The model under review builds one solid part; all positions refer to its coordinate system, in mm. A direction names the side the tool comes from. Give positions to 0.01 mm unless a question says otherwise; leave off trailing zeros. Loops run counter-clockwise (first coordinate to the right, second up) from the corner with the lowest first, then second, coordinate; pieces in that order, holes last. Notation, with made-up numbers: M -15.5,-21.5 L 37.5,-21.5 A12 cw 37.5,-0.5 Z; hole C -31,77 d4. An arc over 180 degrees is marked long. Return JSON: item names as keys, results as strings.
```python
from build123d import *

# Parameters (mm, degrees)
F0_R     = 11
F2_DEPTH = 2.5
F1_R     = 3.1
F1_R_2   = 1.25
F1_R_3   = 1
F3_DEPTH = 2.501
F4_R     = 2.2
F5_DEPTH = 1.8
F6_R     = 6.3
F7_DEPTH = 0.8
F8_DEPTH = 0.8
F9_DEPTH = 3.301


with BuildPart() as f2:
    # F0 (on Front) → F2 (new body)
    with BuildSketch(Plane.XZ):
        Circle(F0_R)
    extrude(amount=F2_DEPTH)

    # F1 (on Front) → F3 (cut, through all)
    with BuildSketch(Plane.XZ):
        Circle(F1_R)
        with Locations((-6.5, 0)):
            Circle(F1_R_2)
        with Locations((-6.363961, 6.363961)):
            Circle(F1_R_3)
        with Locations((-6.363961, -6.363961)):
            Circle(F1_R_3)
        with Locations((6.363961, -6.363961)):
            Circle(F1_R_3)
        with Locations((6.363961, 6.363961)):
            Circle(F1_R_3)
        with Locations((6.5, 0)):
            Circle(F1_R_2)
        with BuildLine():
            ThreePointArc((1.1, -5), (0, -3.9), (-1.1, -5))
            Line((-1.1, -5), (-1.1, -6.133975))
            ThreePointArc((-1.1, -6.133975), (-1.4, -7), (-1.1, -7.866025))
            Line((-1.1, -7.866025), (-1.1, -8.5))
            ThreePointArc((-1.1, -8.5), (0, -9.6), (1.1, -8.5))
            Line((1.1, -8.5), (1.1, -7.866025))
            ThreePointArc((1.1, -7.866025), (1.4, -7), (1.1, -6.133975))
            Line((1.1, -6.133975), (1.1, -5))
        make_face()
        with BuildLine():
            Line((-1.1, 8.5), (-1.1, 7.866025))
            ThreePointArc((-1.1, 7.866025), (-1.4, 7), (-1.1, 6.133975))
            Line((-1.1, 6.133975), (-1.1, 5))
            ThreePointArc((-1.1, 5), (0, 3.9), (1.1, 5))
            Line((1.1, 5), (1.1, 6.133975))
            ThreePointArc((1.1, 6.133975), (1.4, 7), (1.1, 7.866025))
            Line((1.1, 7.866025), (1.1, 8.5))
            ThreePointArc((1.1, 8.5), (0, 9.6), (-1.1, 8.5))
        make_face()
    extrude(amount=F3_DEPTH, mode=Mode.SUBTRACT)

    # F4 (on face) → F5 (cut)
    with BuildSketch(Plane.XZ.offset(2.5)):
        with Locations((-6.5, 0)):
            Circle(F4_R)
        with Locations((6.5, 0)):
            Circle(F4_R)
        with BuildLine():
            Line((1.8, 4.4), (1.8, 5.265065))
            ThreePointArc((1.8, 5.265065), (2.499967, 7.01284), (1.782084, 8.753333))
            ThreePointArc((1.782084, 8.753333), (0, 10.3), (-1.782084, 8.753333))
            ThreePointArc((-1.782084, 8.753333), (-2.499967, 7.01284), (-1.8, 5.265065))
            Line((-1.8, 5.265065), (-1.8, 4.4))
            ThreePointArc((-1.8, 4.4), (-1.634926, 3.646995), (-1.169981, 3.032102))
            ThreePointArc((-1.169981, 3.032102), (0, 3.25), (1.169981, 3.032102))
            ThreePointArc((1.169981, 3.032102), (1.634926, 3.646995), (1.8, 4.4))
        make_face()
        with BuildLine():
            Line((-1.8, -4.4), (-1.8, -5.265065))
            ThreePointArc((-1.8, -5.265065), (-2.499967, -7.01284), (-1.782084, -8.753333))
            ThreePointArc((-1.782084, -8.753333), (0, -10.3), (1.782084, -8.753333))
            ThreePointArc((1.782084, -8.753333), (2.499967, -7.01284), (1.8, -5.265065))
            Line((1.8, -5.265065), (1.8, -4.4))
            ThreePointArc((1.8, -4.4), (1.634926, -3.646995), (1.169981, -3.032102))
            ThreePointArc((1.169981, -3.032102), (0, -3.25), (-1.169981, -3.032102))
            ThreePointArc((-1.169981, -3.032102), (-1.634926, -3.646995), (-1.8, -4.4))
        make_face()
    extrude(amount=-F5_DEPTH, mode=Mode.SUBTRACT)

    # F6 (on face) → F7 (join)
    with BuildSketch(Plane.XZ.offset(2.5)):
        Circle(F6_R)
    extrude(amount=F7_DEPTH)

    # F4 (on face) → F8 (cut)
    with BuildSketch(Plane.XZ.offset(2.5)):
        with Locations((-6.5, 0)):
            Circle(F4_R)
        with Locations((6.5, 0)):
            Circle(F4_R)
        with BuildLine():
            Line((1.8, 4.4), (1.8, 5.265065))
            ThreePointArc((1.8, 5.265065), (2.499967, 7.01284), (1.782084, 8.753333))
            ThreePointArc((1.782084, 8.753333), (0, 10.3), (-1.782084, 8.753333))
            ThreePointArc((-1.782084, 8.753333), (-2.499967, 7.01284), (-1.8, 5.265065))
            Line((-1.8, 5.265065), (-1.8, 4.4))
            ThreePointArc((-1.8, 4.4), (-1.634926, 3.646995), (-1.169981, 3.032102))
            ThreePointArc((-1.169981, 3.032102), (0, 3.25), (1.169981, 3.032102))
            ThreePointArc((1.169981, 3.032102), (1.634926, 3.646995), (1.8, 4.4))
        make_face()
        with BuildLine():
            Line((-1.8, -4.4), (-1.8, -5.265065))
            ThreePointArc((-1.8, -5.265065), (-2.499967, -7.01284), (-1.782084, -8.753333))
            ThreePointArc((-1.782084, -8.753333), (0, -10.3), (1.782084, -8.753333))
            ThreePointArc((1.782084, -8.753333), (2.499967, -7.01284), (1.8, -5.265065))
            Line((1.8, -5.265065), (1.8, -4.4))
            ThreePointArc((1.8, -4.4), (1.634926, -3.646995), (1.169981, -3.032102))
            ThreePointArc((1.169981, -3.032102), (0, -3.25), (-1.169981, -3.032102))
            ThreePointArc((-1.169981, -3.032102), (-1.634926, -3.646995), (-1.8, -4.4))
        make_face()
    extrude(amount=F8_DEPTH, mode=Mode.SUBTRACT)

    # F1 (on Front) → F9 (cut, through all)
    with BuildSketch(Plane.XZ):
        Circle(F1_R)
        with Locations((-6.5, 0)):
            Circle(F1_R_2)
        with Locations((-6.363961, 6.363961)):
            Circle(F1_R_3)
        with Locations((-6.363961, -6.363961)):
            Circle(F1_R_3)
        with Locations((6.363961, -6.363961)):
            Circle(F1_R_3)
        with Locations((6.363961, 6.363961)):
            Circle(F1_R_3)
        with Locations((6.5, 0)):
            Circle(F1_R_2)
        with BuildLine():
            ThreePointArc((1.1, -5), (0, -3.9), (-1.1, -5))
            Line((-1.1, -5), (-1.1, -6.133975))
            ThreePointArc((-1.1, -6.133975), (-1.4, -7), (-1.1, -7.866025))
            Line((-1.1, -7.866025), (-1.1, -8.5))
            ThreePointArc((-1.1, -8.5), (0, -9.6), (1.1, -8.5))
            Line((1.1, -8.5), (1.1, -7.866025))
            ThreePointArc((1.1, -7.866025), (1.4, -7), (1.1, -6.133975))
            Line((1.1, -6.133975), (1.1, -5))
        make_face()
        with BuildLine():
            Line((-1.1, 8.5), (-1.1, 7.866025))
            ThreePointArc((-1.1, 7.866025), (-1.4, 7), (-1.1, 6.133975))
            Line((-1.1, 6.133975), (-1.1, 5))
            ThreePointArc((-1.1, 5), (0, 3.9), (1.1, 5))
            Line((1.1, 5), (1.1, 6.133975))
            ThreePointArc((1.1, 6.133975), (1.4, 7), (1.1, 7.866025))
            Line((1.1, 7.866025), (1.1, 8.5))
            ThreePointArc((1.1, 8.5), (0, 9.6), (-1.1, 8.5))
        make_face()
    extrude(amount=F9_DEPTH, mode=Mode.SUBTRACT)


solid = f2.part
```
1) Consider section D-D on x = 6.5. Write out the cut boundary in (y, z).
From the geometry:
{"outline": "M -2.5,-8.87 L 0,-8.87 L 0,-7.35 L -2.5,-7.35 Z; M -2.5,-5.37 L 0,-5.37 L 0,-1.25 L -0.7,-1.25 L -0.7,-2.2 L -2.5,-2.2 Z; M -2.5,2.2 L -0.7,2.2 L -0.7,1.25 L 0,1.25 L 0,5.37 L -2.5,5.37 Z; M -2.5,7.35 L 0,7.35 L 0,8.87 L -2.5,8.87 Z"}
2) Wall thickness on L1, parallel to X at y = -1.15, z = -1.5; L2, parallel to Z at x = 7.25, y = -0.4; L3, parallel to X at y = -1.2, z = -0.25: over which ranges is each line inside the solid? List them lowest first. Write a range as from..to.
From the geometry:
{"L1": "-10.9..-8.11, -4.89..-2.71, 2.71..4.89, 8.11..10.9", "L2": "-8.27..-6.83, -5.9..-1, 1..5.9, 6.83..8.27", "L3": "-11..-8.69, -4.31..-3.09, 3.09..4.31, 8.69..11"}
3) Consider section B-B on z = -0.5. Write out the cut boundary in (x, y), then the cut area to 3 significant figures.
From the geometry:
{"outline": "M -10.99,-2.5 L -8.64,-2.5 L -8.64,-0.7 L -7.65,-0.7 L -7.65,0 L -10.99,0 Z; M -5.35,-0.7 L -4.36,-0.7 L -4.36,-3.3 L -3.06,-3.3 L -3.06,0 L -5.35,0 Z; M 3.06,-3.3 L 4.36,-3.3 L 4.36,-0.7 L 5.35,-0.7 L 5.35,0 L 3.06,0 Z; M 7.65,-0.7 L 8.64,-0.7 L 8.64,-2.5 L 10.99,-2.5 L 10.99,0 L 7.65,0 Z", "area": "23.1 mm²"}
4) The part is to be moulded in two halves that separate along Z. For faces 4 (the face through (2.3, 0, -2.3)), 5 (the face through (-4.524, -2.894, -4.384)), 6 (the face through (0, -0.3, 3.9)), say which applies: released by +Z, released by -Z, zero draft, split by the parting line, or undercut.
From the geometry:
{"face 4": "zero draft", "face 5": "released by -Z", "face 6": "undercut"}
5) Consider section A-A on x = 0. Write out the cut boundary in (y, z).
From the geometry:
{"outline": "M -3.3,-3.25 L -0.7,-3.25 L -0.7,-3.9 L 0,-3.9 L 0,-3.1 L -3.3,-3.1 Z; M -3.3,3.1 L 0,3.1 L 0,3.9 L -0.7,3.9 L -0.7,3.25 L -3.3,3.25 Z; M -2.5,-11 L 0,-11 L 0,-9.6 L -0.7,-9.6 L -0.7,-10.3 L -2.5,-10.3 Z; M -2.5,10.3 L -0.7,10.3 L -0.7,9.6 L 0,9.6 L 0,11 L -2.5,11 Z"}
6) Insertion check: pin 1 (0.7 mm diameter, centred on y = 0, z = 8, fed in from +X); pin 2 (3.5 mm diameter, centred on x = 0, z = 0, fed in from +Y); pin 3 (1 mm diameter, centred on y = -1.5, z = -5, fed in from -X); pin 4 (1.3 mm diameter, centred on x = 7, z = 0.5, fed in from -Y). Each pin has a flat end and moves straight along its axis. Give the tip position at first contact, or say it passes through.
From the geometry:
{"pin 1": "x = 7.9", "pin 2": "through", "pin 3": "x = -10.04", "pin 4": "y = -0.7"}
7) Tool access review of faces 1 (the face through (-5, -0.7, 0)), 2 (the face through (0, -0.3, -3.9)), 3 (the face through (3, -3.3, 3)): name each direction out of +Z, -Z, +X, -X, +Y, -Y from which nothing blocks a thin tool from reaching the whole face with its end or side.
From the geometry:
{"face 1": "-Y", "face 2": "+Y, -Y", "face 3": "+Z, -Z, +X, -X, -Y"}
8) Consider section C-C on y = -0.3. Count the separate pieces of the cut face and the enclosed holes in it, then the cut area to 3 significant figures.
From the geometry:
{"separate pieces": "1", "enclosed holes": "9", "area": "303 mm²"}
